```python
from build123d import *

# Parameters (mm, degrees)
SKETCH1_W           = 50
SKETCH1_H           = 50
BOSS_EXTRUDE1_DEPTH = 90
CUT_EXTRUDE1_DEPTH  = 19
SKETCH3_W           = 20.00325309
SKETCH3_H           = 20
CUT_EXTRUDE2_DEPTH  = 115.455231423
SKETCH4_R           = 6
CUT_EXTRUDE3_DEPTH  = 66
SKETCH6_R           = 2.75
CUT_EXTRUDE4_DEPTH  = 97.726418315
SKETCH7_R           = 2.75
CUT_EXTRUDE5_DEPTH  = 115.455231423
SKETCH8_R           = 2.75
CUT_EXTRUDE6_DEPTH  = 115.455231423
FILLET1_R           = 3
FILLET2_R           = 1


with BuildPart() as part:
    # Sketch1 → Boss-Extrude1 (new body)
    with BuildSketch(Plane(origin=(0, 0, 0), x_dir=(1, 0, 0), z_dir=(0, 1, 0))):
        with Locations((25, 25)):
            Rectangle(SKETCH1_W, SKETCH1_H)
    extrude(amount=BOSS_EXTRUDE1_DEPTH)

    # Sketch2 → Cut-Extrude1 (cut)
    with BuildSketch(Plane(origin=(0, 90, 0), x_dir=(1, 0, 0), z_dir=(0, 1, 0))):
        Polygon((5, 0), (25, 0), (25, 25), (50, 25), (50, 45), (5, 45), align=None)
    extrude(amount=-CUT_EXTRUDE1_DEPTH, mode=Mode.SUBTRACT)

    # Sketch3 → Cut-Extrude2 (cut, through all)
    with BuildSketch(Plane(origin=(0, 90, 0), x_dir=(1, 0, 0), z_dir=(0, 1, 0))):
        with Locations((39.998373455, 10)):
            Rectangle(SKETCH3_W, SKETCH3_H)
    extrude(amount=-CUT_EXTRUDE2_DEPTH, mode=Mode.SUBTRACT)

    # Sketch4 → Cut-Extrude3 (cut)
    with BuildSketch(Plane.XZ):
        with Locations(Location((14.998373455, -10, 0), (0, 0, 270))):
            Circle(SKETCH4_R)
        with Locations(Location((40, -35, 0), (0, 0, 270))):
            Circle(SKETCH4_R)
        with Locations(Location((14.998373455, -35, 0), (0, 0, 270))):
            Circle(SKETCH4_R)
    extrude(amount=-CUT_EXTRUDE3_DEPTH, mode=Mode.SUBTRACT)

    # Sketch6 → Cut-Extrude4 (cut, through all)
    with BuildSketch(Plane.XZ.offset(-66)):
        with Locations(Location((14.998373455, -10, 0), (0, 0, 270))):
            Circle(SKETCH6_R)
        with Locations(Location((40, -35, 0), (0, 0, 270))):
            Circle(SKETCH6_R)
        with Locations(Location((14.998373455, -35, 0), (0, 0, 270))):
            Circle(SKETCH6_R)
    extrude(amount=-CUT_EXTRUDE4_DEPTH, mode=Mode.SUBTRACT)

    # Sketch7 → Cut-Extrude5 (cut, through all)
    with BuildSketch(Plane.ZY):
        with Locations((-10, 81)):
            Circle(SKETCH7_R)
    extrude(amount=-CUT_EXTRUDE5_DEPTH, mode=Mode.SUBTRACT)

    # Sketch8 → Cut-Extrude6 (cut, through all)
    with BuildSketch(Plane(origin=(0, 0, -50), x_dir=(-1, 0, 0), z_dir=(0, 0, -1))):
        with Locations((-40, 81)):
            Circle(SKETCH8_R)
    extrude(amount=-CUT_EXTRUDE6_DEPTH, mode=Mode.SUBTRACT)

    # Fillet1
    fillet1_edges = [part.edges().sort_by_distance(p)[0] for p in [
        (29.99674691, 45, -20),
        (0, 45, -50),
    ]]
    fillet(fillet1_edges, radius=FILLET1_R)

    # Fillet2
    fillet2_edges = [part.edges().sort_by_distance(p)[0] for p in [
        (30.875426566, 90, -19.121320344),
        (26.5, 90, -50),
        (41.498373455, 90, -20),
        (29.99674691, 90, -8.5),
        (0, 90, -23.5),
        (0.878679656, 90, -49.121320344),
    ]]
    fillet(fillet2_edges, radius=FILLET2_R)


solid = part.part
```
Can you work these out from the model? Positions are in its coordinate system, mm. A direction names the side the tool comes from. Coordinates: 2 decimals unless noted, no trailing zeros. Order: outer loops, then holes, each group sorted by start corner. A loop starts at its lowest first (then second) coordinate and runs counter-clockwise, first axis right, second up.
1. If we section it at B-B (y = 81): Give the number of separate pieces and of enclosed holes in the cut face, then the cut area to 3 significant figures.
2. I need wall thicknesses on line 1 (X direction, y = 69, z = -35); line 2 (X direction, y = 17, z = -35); line 3 (Z direction, x = 14.5, y = 54.5). Which ranges of each line are inside material? Lowest first, please.
3. If we section it at C-C (z = -10): Please give me the cut outline in (x, y).
4. If we section it at A-A (z = -35): Please give me the cut outline in (x, y).
5. I'm going to push flat-ended pins straight in: pin 1 (5 mm diameter, centred on y = 63.5, z = -5, fed in from +X); pin 2 (5.5 mm diameter, centred on y = 78, z = -15, fed in from +X); pin 3 (4.5 mm diameter, centred on x = 15, z = -10, fed in from +Y); pin 4 (8 mm diameter, centred on x = 40, y = 34, fed in from +Z). Where does each tip first touch, or does it pass through?
6. If we section it at D-D (x = 24): Please give me the cut outline in (y, z).
7. Thinking about a two-plate mould opening in Y: for faces 6 (the face through (25, 82.744, -12.325)), 7 (the face through (19, 0, -25)), 8 (the face through (42.747, 81.121, -47.535)), which applies, +Y half, -Y half, draft (parallel to the pull), parting line (faces both ways), or undercut?
8. For faces 1 (the face through (26, 44, -50)), 2 (the face through (28, 81, -45)), 3 (the face through (17.725, 68.465, -9.642)), 4 (the face through (29.997, 45, -8)), 5 (the face through (36.35, 32.54, -30.24)), which set-ups out of +Z, -Z, +X, -X, +Y, -Y let a thin tool reach every point of the face, with its end or its side?
Entries:
1. separate pieces: 6
1. enclosed holes: 0
1. area: 590 mm2
2. line 1: x = 0 to 12.25, 17.75 to 37.25, 42.75 to 50
2. line 2: x = 0 to 9, 21 to 34, 46 to 50
2. line 3: z = -50 to -40.98, -29.02 to -15.98, -4.02 to 0
3. outline: (0, 0) - (9, 0) - (9, 66) - (12.25, 66) - (12.25, 71) - (5, 71) - (5, 78.25) - (0, 78.25) - close; (0, 83.75) - (5, 83.75) - (5, 90) - (1, 90) arc R1 ccw to (0, 89) - close; (17.75, 66) - (21, 66) - (21, 0) - (30, 0) - (30, 78.25) - (25, 78.25) - (25, 71) - (17.75, 71) - close; (25, 83.75) - (30, 83.75) - (30, 89) arc R1 ccw to (29, 90) - (25, 90) - close
4. outline: (0, 0) - (9, 0) - (9, 66) - (12.25, 66) - (12.25, 71) - (5, 71) - (5, 90) - (1, 90) arc R1 ccw to (0, 89) - close; (17.75, 66) - (21, 66) - (21, 0) - (34, 0) - (34, 66) - (37.25, 66) - (37.25, 71) - (17.75, 71) - close; (42.75, 66) - (46, 66) - (46, 0) - (50, 0) - (50, 71) - (42.75, 71) - close
5. pin 1: stops at x = 30
5. pin 2: stops at x = 30.09
5. pin 3: passes through
5. pin 4: stops at z = -20
6. outline: (0, -50) - (89, -50) arc R1 ccw to (90, -49) - (90, -45) - (71, -45) - (71, 0) - (0, 0) - close
7. face 6: draft
7. face 7: -Y half
7. face 8: undercut
8. face 1: -Z, +X, -X, +Y, -Y
8. face 2: +X, +Y
8. face 3: +Y, -Y
8. face 4: +Z, +X, +Y, -Y
8. face 5: -Y
